CAD build for the part. Positions are in the model's coordinates, mm. Coordinates: 2 decimals unless noted, no trailing zeros. Loops run counter-clockwise (first coordinate to the right, second up) from the corner with the lowest first, then second, coordinate; pieces in that order, holes last. Notation, with made-up numbers: (67.5, 9) - (98.5, 9) arc R21 ccw to (98.5, 38) - close; hole circle Ø5 at (-5, -5.75). An arc over 180 degrees is marked (long way). Put each result on its own line as item: value.
```python
from build123d import *

# Parameters (mm, degrees)
EXTRUDE1_DEPTH     = 17.78
CUT_EXTRUDE1_DEPTH = 5.08
SKETCH4_W          = 25.7175
SKETCH4_H          = 413.5501
CUT_EXTRUDE2_DEPTH = 11.43
SKETCH5_R          = 15.08125
SKETCH5_R_2        = 2.36855
SKETCH5_R_3        = 1.5875
CUT_EXTRUDE3_DEPTH = 17.78


with BuildPart() as part:
    # Sketch2 → Extrude1 (new body)
    with BuildSketch(Plane.XY):
        Polygon((10946.341666666, -4853.78125), (10946.341666666, -5248.275), (10951.104166666, -5253.0375), (12249.679166666, -5253.0375), (12254.441666666, -5248.275), (12254.441666666, -4722.091838581), (12082.991666666, -4722.091838581), align=None)
    extrude(amount=-EXTRUDE1_DEPTH)

    # Sketch3 → Cut-Extrude1 (cut)
    with BuildSketch(Plane.XY):
        with BuildLine():
            Line((10943.166666666, -5225.7325), (10943.166666666, -5243.5125))
            Line((10943.166666666, -5243.5125), (12236.661666666, -5243.5125))
            Line((12236.661666666, -5243.5125), (12236.661666666, -5256.2125))
            Line((12236.661666666, -5256.2125), (12257.616666666, -5256.2125))
            Line((12257.616666666, -5256.2125), (12257.616666666, -4715.591300541))
            Line((12257.616666666, -4715.591300541), (12236.661666666, -4715.591300541))
            Line((12236.661666666, -4715.591300541), (12236.661666666, -5225.7325))
            Line((12236.661666666, -5225.7325), (11824.335, -5225.7325))
            Line((11824.335, -5225.7325), (11824.335, -5146.402628061))
            ThreePointArc((11824.335, -5146.402628061), (11824.335, -5141.9125), (11819.844871939, -5141.9125))
            Line((11819.844871939, -5141.9125), (11811.045128061, -5141.9125))
            ThreePointArc((11811.045128061, -5141.9125), (11806.555, -5141.912499999), (11806.554999999, -5146.402628059))
            Line((11806.554999999, -5146.402628059), (11806.555, -5225.7325))
            Line((11806.555, -5225.7325), (11394.228333334, -5225.7325))
            Line((11394.228333334, -5225.7325), (11394.228333334, -5146.402628061))
            ThreePointArc((11394.228333334, -5146.402628061), (11394.228333334, -5141.912499999), (11389.738205272, -5141.912499999))
            Line((11389.738205272, -5141.912499999), (11380.938461393, -5141.912499999))
            ThreePointArc((11380.938461393, -5141.912499999), (11376.448333333, -5141.9125), (11376.448333334, -5146.402628061))
            Line((11376.448333334, -5146.402628061), (11376.448333334, -5225.7325))
            Line((11376.448333334, -5225.7325), (10943.166666666, -5225.7325))
        make_face()
    extrude(amount=-CUT_EXTRUDE1_DEPTH, mode=Mode.SUBTRACT)

    # Sketch4 → Cut-Extrude2 (cut)
    with BuildSketch(Plane.XY):
        with Locations((10951.262916666, -5051.02495)):
            Rectangle(SKETCH4_W, SKETCH4_H)
    extrude(amount=-CUT_EXTRUDE2_DEPTH, mode=Mode.SUBTRACT)

    # Sketch5 → Cut-Extrude3 (cut)
    with BuildSketch(Plane.XY):
        with Locations((11037.231463428, -4887.549352662)):
            Circle(SKETCH5_R)
        with Locations((10979.132281191, -4867.008218481)):
            Circle(SKETCH5_R_2)
        with Locations((10955.231666666, -4929.98125)):
            Circle(SKETCH5_R_3)
        with Locations((10955.231666666, -5031.58125)):
            Circle(SKETCH5_R_3)
        with Locations((11003.809166666, -5062.5375)):
            Circle(SKETCH5_R_3)
        with Locations((11003.809166666, -5119.6875)):
            Circle(SKETCH5_R_3)
        with Locations((11003.809166666, -5176.8375)):
            Circle(SKETCH5_R_3)
        with Locations((11251.141666666, -5234.6225)):
            Circle(SKETCH5_R_3)
        with Locations((11098.741666666, -5234.6225)):
            Circle(SKETCH5_R_3)
        with Locations((11385.338333334, -5160.9625)):
            Circle(SKETCH5_R_3)
        with Locations((11385.338333334, -5193.9825)):
            Circle(SKETCH5_R_3)
        with Locations((11530.541666666, -5234.6225)):
            Circle(SKETCH5_R_3)
        with Locations((11682.941666666, -5234.6225)):
            Circle(SKETCH5_R_3)
        with Locations((11815.445, -5160.9625)):
            Circle(SKETCH5_R_3)
        with Locations((11815.445, -5193.9825)):
            Circle(SKETCH5_R_3)
        with Locations((11962.341666666, -5234.6225)):
            Circle(SKETCH5_R_3)
        with Locations((12114.741666666, -5234.6225)):
            Circle(SKETCH5_R_3)
        with Locations((12196.974166666, -5202.2375)):
            Circle(SKETCH5_R_3)
        with Locations((12196.974166666, -5145.0875)):
            Circle(SKETCH5_R_3)
        with Locations((12245.551666666, -5134.504166666)):
            Circle(SKETCH5_R_3)
        with Locations((12196.974166666, -5087.9375)):
            Circle(SKETCH5_R_3)
        with Locations((12245.551666666, -5015.970833334)):
            Circle(SKETCH5_R_3)
        with Locations((12245.551666666, -4897.4375)):
            Circle(SKETCH5_R_3)
        with Locations((12245.551666666, -4778.904166666)):
            Circle(SKETCH5_R_3)
        with Locations((12106.652677233, -4736.376540025)):
            Circle(SKETCH5_R_2)
    extrude(amount=-CUT_EXTRUDE3_DEPTH, mode=Mode.SUBTRACT)


solid = part.part
```
Q1. Mould opens along X. For faces 1 (the flat face through (11522.623, -4787.015, -8.766)), 2 (the cylindrical face through (11026.116, -4877.357, -8.766)), 3 (the flat face through (11591, -4970, 0)) say: +X half, -X half, draft (parallel to the pull), parting line (faces both ways), or undercut.
Determined:
face 1: -X half
face 2: undercut
face 3: draft
Q2. Pin check, flat tips, straight feed: pin 1 Ø2.5 at (x, y) = (12196.97, -5087.94) entering from +Z; pin 2 Ø4 at (x, y) = (12245.55, -5134.5) entering from +Z; pin 3 Ø2.5 at (y, z) = (-5169, -3.5) entering from -X. Stop position of each tip, or through.
Determined:
pin 1: through
pin 2: z = -5.08
pin 3: x = 10964.12
Q3. Slice it at A-A, the plane x = 11138. Give the cut face in (y, z).
Determined:
outline: (-5253.04, -17.78) - (-4831.58, -17.78) - (-4831.58, 0) - (-5225.73, 0) - (-5225.73, -5.08) - (-5243.51, -5.08) - (-5243.51, 0) - (-5253.04, 0) - close
Q4. Slice it at C-C, the plane x = 11753.5. Give the cut face in (y, z).
Determined:
outline: (-5253.04, -17.78) - (-4760.27, -17.78) - (-4760.27, 0) - (-5225.73, 0) - (-5225.73, -5.08) - (-5243.51, -5.08) - (-5243.51, 0) - (-5253.04, 0) - close
Q5. Wall check: L1, parallel to Y at x = 12099.5, z = -4; L2, parallel to X at y = -5203, z = -17; L3, parallel to X at y = -5196, z = -2.25 (3 decimals). Give the ranges that are in metal, low to high. Write a range as from..to.
Determined:
L1: -5253.04..-5243.51, -5225.73..-4722.09
L2: 10946.34..12195.58, 12198.37..12254.44
L3: 10964.122..11376.448, 11394.228..11806.555, 11824.335..12236.662
Q6. Slice it at B-B, the plane y = -4818.5. Give the cut face in (x, z), then the cut area to 3 significant figures.
Determined:
outline: (11250.86, -17.78) - (12254.44, -17.78) - (12254.44, -5.08) - (12236.66, -5.08) - (12236.66, 0) - (11250.86, 0) - close
area: 17,800 mm2
